For this review, take the finished solid that the model builds, in its own axes (mm). Face numbers are marked on the shaded views. Give positions to 0.01 mm unless a question says otherwise; leave off trailing zeros. Loops run counter-clockwise (first coordinate to the right, second up) from the corner with the lowest first, then second, coordinate; pieces in that order, holes last. Notation, with made-up numbers: (-35.75, -7.5) - (8.25, -7.5) arc R17 ccw to (8.25, 11.5) - close; hole circle Ø6 at (53, 45). An arc over 180 degrees is marked (long way). Answer in a Markdown table with one row per item.
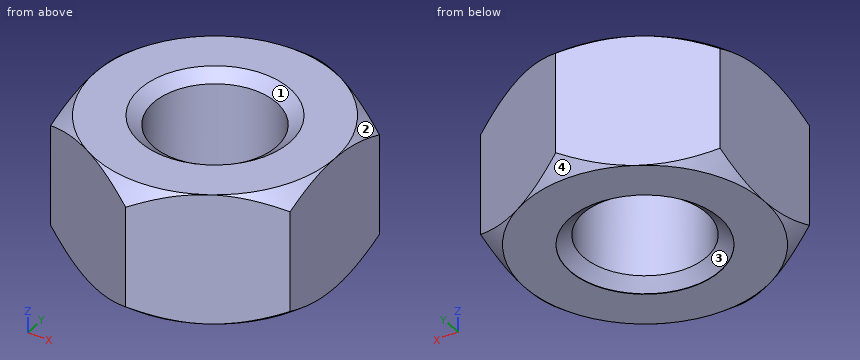
```python
from build123d import *

# Parameters (mm, degrees)
BASENUT_START = -6.9342
BASENUTSKE_R  = 3.2639
BASENUT_DEPTH = 6.9342


# Read off the part's stored shape, not the designer's step: ThreadSchematic
with BuildPart() as part:
    # BaseNutSke → BaseNut (new body)
    with BuildSketch(Plane.XY.offset(BASENUT_START)):
        Polygon((6.35, 3.666174209), (6.35, -3.666174209), (0, -7.332348419), (-6.35, -3.666174209), (-6.35, 3.666174209), (0, 7.332348419), align=None)
        Circle(BASENUTSKE_R, mode=Mode.SUBTRACT)
    extrude(amount=BASENUT_DEPTH)

    # Sketch5 (on Front Plane) → EndChamfer (revolve, cut)
    with BuildSketch(Plane.XY):
        Polygon((6.9088, 3.96875), (6.365904588, 3.193415), (6.9596, 3.193415), (6.9596, 3.96875), align=None)
    revolve(axis=Axis((6.9088, 3.96875, 0), (-0.5735764363510457, -0.819152044288992, 0)), mode=Mode.SUBTRACT)

    # Sketch3 → Double-Chamfer (revolve, cut)
    with BuildSketch(Plane(origin=(0, 0, 0), x_dir=(0, 0, -1), z_dir=(1, 0, 0))):
        Polygon((6.9342, 6.35), (6.14045, 7.332348419), (6.14045, 20.032348419), (19.6342, 20.032348419), (19.6342, 6.35), align=None)
        Polygon((0.79375, 20.032348419), (-12.7, 20.032348419), (-12.7, 6.35), (0, 6.35), (0.79375, 7.332348419), align=None)
    revolve(axis=Axis((0, 0, 0), (0, 0, -1)), mode=Mode.SUBTRACT)

    # ThreadSchematic outline → ThreadSchematic (revolve, cut)
    with BuildSketch(Plane.XZ):
        Polygon((3.2639, 0), (3.2639, -0.493541283), (3.96875, 0), align=None)
        Polygon((3.96875, -6.9088), (3.2639, -6.415258717), (3.2639, -6.9342), (3.96875, -6.9342), align=None)
    revolve(axis=Axis((0, 0, 0), (0, 0, 1)), mode=Mode.SUBTRACT)


solid = part.part
```
1. Wall thickness on line 1 (Y direction, x = -1, z = -3.25) (3 decimals); line 2 (Y direction, x = -0.75, z = -4.25); line 3 (X direction, y = 0, z = -6.5): over which ranges is each line inside the solid? List them lowest first. Write a range as [from, to].
Values:
| item | result |
|---|---|
| line 1 | y = [-6.755, -3.107], [3.107, 6.755] |
| line 2 | y = [-6.9, -3.18], [3.18, 6.9] |
| line 3 | x = [-6.35, -3.38], [3.38, 6.35] |
2. Clearance check with flat-ended pins moving along their axes: pin 1 (6 mm diameter, centred on x = -2, y = 1, fed in from +Z); pin 2 (1 mm diameter, centred on y = -4.5, z = -6, fed in from -X). State where each tip first meets the part, or that it passes through.
Values:
| item | result |
|---|---|
| pin 1 | stops at z = 0 |
| pin 2 | stops at x = -5.77 |
3. Mouldability with a two-part tool opening along X and no side actions: class the marked faces 1, 2, 3 and 4 as released by +X, released by -X, zero draft, split by the parting line, or undercut.
Values:
| item | result |
|---|---|
| face 1 | undercut |
| face 2 | released by +X |
| face 3 | undercut |
| face 4 | split by the parting line |
4. We need section A-A, the plane z = -3.75. Give the boundary of the cut face in (x, y), and give its area (3 significant figures).
Values:
| item | result |
|---|---|
| outline | (-6.35, -3.67) - (0, -7.33) - (6.35, -3.67) - (6.35, 3.67) - (0, 7.33) - (-6.35, 3.67) - close; hole circle Ø6.53 at (0, 0) |
| area | 106 mm^2 |
